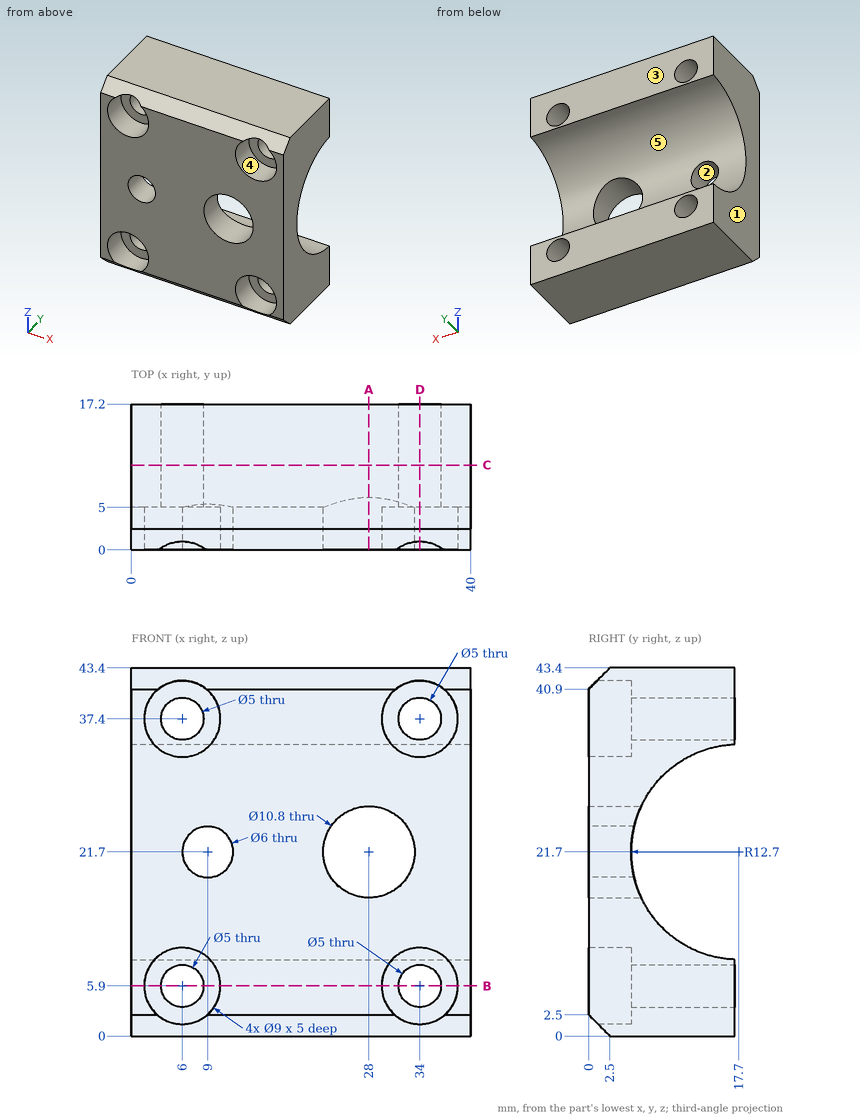
Source: three-view drawing plus pictorial views. Frame: mm from the lowest corner of the part. A direction names the side the tool comes from. Give positions to 0.01 mm unless a question says otherwise; leave off trailing zeros. Order: outer loops, then holes, each group sorted by start corner. A loop starts at its lowest first (then second) coordinate and runs counter-clockwise, first axis right, second up. Notation, with made-up numbers: M 39,-12 L 95,-12 A22 cw 95,19 Z; hole C 37.5,72 d6. An arc over 180 degrees is marked long. Return JSON: item names as keys, results as strings.
Item 1: Cut plane B-B (z = 5.9). Return loops of the section in (x, y), then the cut area to 3 significant figures.
Solutions:
{"outline": "M 0,0 L 1.5,0 L 1.5,5 L 3.5,5 L 3.5,17.2 L 0,17.2 Z; M 8.5,5 L 10.5,5 L 10.5,0 L 29.5,0 L 29.5,5 L 31.5,5 L 31.5,17.2 L 8.5,17.2 Z; M 36.5,5 L 38.5,5 L 38.5,0 L 40,0 L 40,17.2 L 36.5,17.2 Z", "area": "476 mm^2"}
Item 2: Pull-direction query (X, two-part tool) for the marked faces 1, 2 and 3; classes: +X half, -X half, draft (parallel to the pull), parting line (faces both ways), or undercut.
Solutions:
{"face 1": "-X half", "face 2": "undercut", "face 3": "draft"}
Item 3: Ray query, probe 1 along X at (y, z) = (2.65, 5.9); probe 2 along Z at (x, y) = (6, 8.5) (3 decimals); probe 3 along X at (y, z) = (6.5, 36). Return the intervals inside material, ascending.
Solutions:
{"probe 1": "0 to 1.5, 10.5 to 29.5, 38.5 to 40", "probe 2": "0 to 3.4, 8.4 to 12.945, 30.455 to 34.9, 39.9 to 43.4", "probe 3": "0 to 3.93, 8.07 to 31.93, 36.07 to 40"}
Item 4: Access query for the marked faces 4 and 5. Directions: +Z, -Z, +X, -X, +Y, -Y. A direction counts if a zero-diameter tool reaches every point of the face in a straight line with its end or side. Return the directions, or none.
Solutions:
{"face 4": "-Y", "face 5": "+X, -X, +Y"}
Item 5: Cut plane A-A (x = 28). Return loops of the section in (y, z), then the cut area to 3 significant figures.
Solutions:
{"outline": "M 0,2.5 L 2.5,0 L 17.2,0 L 17.2,9.01 A12.7 cw 6.21,16.3 L 0,16.3 Z; M 0,27.1 L 6.21,27.1 A12.7 cw 17.2,34.39 L 17.2,43.4 L 2.5,43.4 L 0,40.9 Z", "area": "441 mm^2"}
Item 6: Cut plane C-C (y = 10). Return loops of the section in (x, z).
Solutions:
{"outline": "M 0,0 L 40,0 L 40,11.6 L 0,11.6 Z; M 0,31.8 L 40,31.8 L 40,43.4 L 0,43.4 Z; hole C 6,5.9 d5; hole C 6,37.4 d5; hole C 34,5.9 d5; hole C 34,37.4 d5"}
Item 7: First-contact query: P1, Ø6.5, axis at x = 34, z = 37.4, coming from the -Y side; P2, Ø1, axis at x = 17.5, z = 21, coming from the +Y side; P3, Ø8, axis at x = 25, z = 20.5, coming from the +Y side. Flat tips, straight axial feed; report the tip coordinate or a pass-through.
Solutions:
{"P1": "y = 5", "P2": "y = 5.06", "P3": "y = 6.11"}
Item 8: Cut plane D-D (x = 34). Return loops of the section in (y, z), then the cut area to 3 significant figures.
Solutions:
{"outline": "M 0,10.4 L 5,10.4 L 5,8.4 L 17.2,8.4 L 17.2,9.01 A12.7 cw 17.2,34.39 L 17.2,34.9 L 5,34.9 L 5,32.9 L 0,32.9 Z; M 1,41.9 L 5,41.9 L 5,39.9 L 17.2,39.9 L 17.2,43.4 L 2.5,43.4 Z; M 1.1,1.4 L 2.5,0 L 17.2,0 L 17.2,3.4 L 5,3.4 L 5,1.4 Z", "area": "289 mm^2"}
